from build123d import *

# Parameters (mm, degrees)
BOSS_EXTRUDE1_DEPTH = 2
BOSS_EXTRUDE2_DEPTH = 9.2
CUT_EXTRUDE1_REACH  = 23.032


with BuildPart() as part:
    # Sketch1 → Boss-Extrude1 (new body)
    with BuildSketch(Plane.XY):
        Polygon((3, -2.075), (13, -2.075), (13, -7.125), (18, -7.125), (18, -2.075), (18, 2.075), (5.25, 2.075), (5.25, 3.075), (-5.25, 3.075), (-5.25, 2.075), (-18, 2.075), (-18, -2.075), (-18, -7.125), (-13, -7.125), (-13, -2.075), (-3, -2.075), (-3, -7.125), (3, -7.125), align=None)
    extrude(amount=BOSS_EXTRUDE1_DEPTH)

    # Sketch2 → Boss-Extrude2 (add)
    with BuildSketch(Plane(origin=(0, 2.075, 0), x_dir=(1, 0, 0), z_dir=(0, 1, 0))):
        Polygon((-18, 0), (-18.806783424, -2), (-18, -2), align=None)
        Polygon((18, 0), (18, -2), (18.806783424, -2), align=None)
    extrude(amount=-BOSS_EXTRUDE2_DEPTH)

    # Sketch3 → Cut-Extrude1 (cut, up to next)
    with BuildSketch(Plane(origin=(0, 2.075, 0), x_dir=(1, 0, 0), z_dir=(0, 1, 0)), mode=Mode.PRIVATE) as cut_extrude1_sk1:
        with BuildLine():
            Line((-18.519101852, -1.286843127), (-18.806783424, -2))
            Line((-18.806783424, -2), (-17.298843892, -2))
            ThreePointArc((-17.298843892, -2), (-17.912522366, -1.649494979), (-18.519101852, -1.286843127))
        make_face()
    cut_extrude1_tool1 = extrude(cut_extrude1_sk1.sketch, amount=-CUT_EXTRUDE1_REACH, mode=Mode.PRIVATE) & part.part
    # Sketch3 → Cut-Extrude1 (cut, up to next)
    with BuildSketch(Plane(origin=(0, 2.075, 0), x_dir=(1, 0, 0), z_dir=(0, 1, 0)), mode=Mode.PRIVATE) as cut_extrude1_sk2:
        with BuildLine():
            Line((18.806783424, -2), (17.298843892, -2))
            ThreePointArc((17.298843892, -2), (17.912522366, -1.649494979), (18.519101852, -1.286843127))
            Line((18.519101852, -1.286843127), (18.806783424, -2))
        make_face()
    cut_extrude1_tool2 = extrude(cut_extrude1_sk2.sketch, amount=-CUT_EXTRUDE1_REACH, mode=Mode.PRIVATE) & part.part
    add(cut_extrude1_tool1.solids().sort_by_distance((-18.211961, 2.075, 1.763734))[0], mode=Mode.SUBTRACT)
    add(cut_extrude1_tool2.solids().sort_by_distance((18.211961, 2.075, 1.763734))[0], mode=Mode.SUBTRACT)


solid = part.part
Geometry check sheet. Reference: the model listing, model coordinates, mm. A direction names the side the tool comes from. Coordinates: 2 decimals unless noted, no trailing zeros. Order: outer loops, then holes, each group sorted by start corner. A loop starts at its lowest first (then second) coordinate and runs counter-clockwise, first axis right, second up. Notation, with made-up numbers: (-31, 80) -> (-10, 80) arc R16 ccw to (-10, 98) -> close; hole circle Ø5 at (-28.5, 69.5). An arc over 180 degrees is marked (long way). Use a Markdown table: item, result. Add a question column.
1. Set-up check for faces 1 (the face through (12, 2.075, 1)), 2 (the face through (-12, 2.075, 1)), 3 (the face through (-13, -5, 1)), 4 (the face through (0, -1, 2)): record each of +Z, -Z, +X, -X, +Y, -Y from which the full face is reachable in a straight line by a thin tool's end or side.
2. Go/stop test with flat-tipped pins: pin 1 Ø1.5 at (x, y) = (-7.5, -3) entering from +Z; pin 2 Ø0.6 at (x, z) = (10, 1) entering from +Y (3 decimals); pin 3 Ø1 at (y, z) = (-4, 0.5) entering from -X; pin 4 Ø0.8 at (y, z) = (3, 1) entering from -X. Record where each tip stops, or that it passes through.
3. Material ranges on L1, parallel to X at y = -4, z = 1.6; L2, parallel to X at y = -5, z = 1.1; L3, parallel to Y at x = -14, z = 1.5 (3 decimals), recorded low to high.
4. Cross-section at A-A (y = -3.5). Enter the section's corners in (x, z), and give its area (3 significant figures).
5. Mould release check, pull along X, two halves, no side actions. Record for faces 5 (the face through (17.904, -2.461, 1.654)), 6 (the face through (-3, -5, 1)), 7 (the face through (-18.256, -2.461, 0.634)): pulls with the +X half, pulls with the -X half, needs draft (parallel to the pull), parting line crosses it, or undercut.
6. Cross-section at D-D (x = 4.5). Enter the section's corners in (y, z) (3 decimals), and give its area (3 significant figures).
7. Cross-section at C-C (z = 0.4). Enter the section's corners in (x, y) (3 decimals).
8. Cross-section at B-B (x = -14). Enter the section's corners in (y, z) (3 decimals), and give its area (3 significant figures).
Filled sheet:
| question | item | result |
|---|---|---|
| 1 | face 1 | +Z, -Z, +X, +Y |
| 1 | face 2 | +Z, -Z, -X, +Y |
| 1 | face 3 | +Z, -Z, -Y |
| 1 | face 4 | +Z, +X, -X, +Y, -Y |
| 2 | pin 1 | through |
| 2 | pin 2 | y = 2.075 |
| 2 | pin 3 | x = -18.4 |
| 2 | pin 4 | x = -5.25 |
| 3 | L1 | -18 to -13, -3 to 3, 13 to 18 |
| 3 | L2 | -18.44 to -13, -3 to 3, 13 to 18.44 |
| 3 | L3 | -7.125 to 2.075 |
| 4 | outline | (-18.52, 1.29) -> (-18, 0) -> (-13, 0) -> (-13, 2) -> (-17.3, 2) arc R35.5 ccw to start; (-3, 0) -> (3, 0) -> (3, 2) -> (-3, 2) -> close; (13, 0) -> (18, 0) -> (18.52, 1.29) arc R35.5 ccw to (17.3, 2) -> (13, 2) -> close |
| 4 | area | 32.6 mm2 |
| 5 | face 5 | pulls with the +X half |
| 5 | face 6 | undercut |
| 5 | face 7 | pulls with the -X half |
| 6 | outline | (-2.075, 0) -> (3.075, 0) -> (3.075, 2) -> (-2.075, 2) -> close |
| 6 | area | 10.3 mm2 |
| 7 | outline | (-18.161, -7.125) -> (-13, -7.125) -> (-13, -2.075) -> (-3, -2.075) -> (-3, -7.125) -> (3, -7.125) -> (3, -2.075) -> (13, -2.075) -> (13, -7.125) -> (18.161, -7.125) -> (18.161, 2.075) -> (5.25, 2.075) -> (5.25, 3.075) -> (-5.25, 3.075) -> (-5.25, 2.075) -> (-18.161, 2.075) -> close |
| 8 | outline | (-7.125, 0) -> (2.075, 0) -> (2.075, 2) -> (-7.125, 2) -> close |
| 8 | area | 18.4 mm2 |
